Geometry check sheet. Reference: the model listing, model coordinates, mm. A direction names the side the tool comes from. Round coordinates to 2 decimals unless told otherwise and drop trailing zeros. Order: outer loops, then holes, each group sorted by start corner. A loop starts at its lowest first (then second) coordinate and runs counter-clockwise, first axis right, second up. Notation, with made-up numbers: M 20,6 L 74,6 A32 ccw 74,44 Z; hole C 76,67.5 d5. An arc over 180 degrees is marked long. Return JSON: item names as keys, results as strings. Group by question number.
Autodesk Inventor part; units mm, degrees
ref_plane "XZ Plane" through (0, 0, 0) normal (0, 1, 0) x (-1, 0, 0)
ref_plane "XY Plane" through (0, 0, 0) normal (0, 0, 1) x (1, 0, 0)
sketch "Náčrt1" plane through (0, 0, 0) normal (0, 0, 1) x (1, 0, 0)
  line L0 (0, 19.6) -> (0, -19.6)
  line L1 (-19.6, 0) -> (19.6, 0)
  circle A0 centre (0, 0) radius 14
  dimension "d0" = 28
extrude "Vysunutí1" add sketch "Náčrt1" along normal blind 19.2
fillet "Zaoblení1" radius 1 1 edges at (-14, 0, 19.2)
sketch "Náčrt2" plane through (0, 0, 0) normal (0, 0, -1) x (-1, 0, 0)
  line L0 (-7.25, 11) -> (7.25, 11)
  line L1 (7.25, 11) -> (7.25, 17)
  line L2 (7.25, 17) -> (-7.25, 17)
  line L3 (-7.25, 17) -> (-7.25, 11)
  circle A0 centre (0, 0) radius 14
  line L4 (-7.25, 11) -> (7.25, 17) construction
  line L5 (7.25, 11) -> (-7.25, 17) construction
  circle A1 centre (0, 0) radius 15.5
  line L6 (-8.6, 12.8953) -> (-8.6, 11.0472)
  line L7 (8.6, 12.8953) -> (8.6, 11.0472)
  point P0 (0, 14)
  point P1 (0, 14)
  point P2 (7.25, 13.6999)
  point P3 (-7.25, 13.6999)
  dimension "d4" = 14.5
  dimension "d5" = 31
  dimension "d6" = 17.2
  dimension "d7" = 1.35
  dimension "d8" = 1.35
  dimension "d9" = 1.5
extrude "Vysunutí2" add sketch "Náčrt2" against normal blind 16.5 contours A0 L6 A1 L3 | L3 A1 L1 A0 | L1 A1 L7 A0 | L3 L2 L1 A1
sketch "Náčrt3" plane through (0, 0, 0) normal (0, 0, -1) x (-1, 0, 0)
  circle A0 centre (0, -8) radius 4.6
  line L0 (0, -12.6) -> (0, -14) construction
  arc A1 (-8.6, 11.0472) -> (8.6, 11.0472) centre (0, 0) ccw construction
  dimension "d12" = 9.2
  dimension "d14" = 1.4
extrude "Vysunutí3" add sketch "Náčrt3" along normal blind 1.7
sketch "Náčrt4" plane through (0, -8, -1.7) normal (0, 0, -1) x (-1, 0, 0)
  circle A0 centre (0, 0) radius 4.6
  circle A1 centre (0, 0) radius 2.5
  line L0 (-1.475, 2.0185) -> (-1.475, -2.0185)
  line L1 (1.475, 2.0185) -> (1.475, -2.0185)
  point P0 (0, 8)
  dimension "d17" = 5
  dimension "d18" = 2.95
extrude "Vysunutí4" add sketch "Náčrt4" along normal blind 8 contours L1 A1 L0
sketch "Náčrt5" plane through (0, -8, -1.7) normal (0, 0, -1) x (-1, 0, 0)
  arc A0 (1.475, 2.0185) -> (-1.475, 2.0185) centre (0, 0) ccw
  circle A1 centre (0, 0) radius 2.5
  point P0 (0, 8)
  point P1 (-1.475, 2.0185)
  point P2 (1.475, 2.0185)
extrude "Vysunutí5" add sketch "Náčrt5" along normal blind 2
sketch "Sketch6" plane through (0, 0, 0) normal (0, 0, -1) x (-1, 0, 0)
  line L0 (-17.5, 0) -> (17.5, 0) construction
  line L1 (-17.5, -3.5) -> (17.5, -3.5)
  line L2 (17.5, 3.5) -> (-17.5, 3.5)
  arc A0 (-17.5, 3.5) -> (-17.5, -3.5) centre (-17.5, 0) ccw
  arc A1 (17.5, -3.5) -> (17.5, 3.5) centre (17.5, 0) ccw
  circle A2 centre (-17.5, 0) radius 2.1
  circle A3 centre (17.5, 0) radius 2.1
  point P0 (0, 0)
  dimension "d23" = 4.2
  dimension "d24" = 35
  dimension "d25" = 7
extrude "Extrusion6" add sketch "Sketch6" against normal blind 1
equation "\"d7\" = d8"
properties part number "Motor"
Q1. Section check B-B on z = 0.5. Record the cut outline in (x, y), plus the area to 3 significant figures.
Q2. Set-up check for faces 1 (the face through (15.6, -3.5, 0.5)), 2 (the face through (-15.6, 3.5, 0.5)), 3 (the face through (2, -8, -3.7)), 4 (the face through (-1.34, -10.11, -4.76)), 5 (the face through (8.6, 12, 8)): record each of +Z, -Z, +X, -X, +Y, -Y from which the full face is reachable in a straight line by a thin tool's end or side.
Q3. Material ranges on line 1 along Y through (x, z) = (17.5, 0.7); line 2 along X through (y, z) = (-10, -4.5) (3 decimals); line 3 along Z through (x, y) = (2.5, -2), recorded low to high.
Q4. Section check C-C on x = 0. Record the cut outline in (y, z), plus the area to 3 significant figures.
Q5. Section check A-A on y = 0. Record the cut outline in (x, z).
Q6. Section check D-D on z = 17.25. Record the cut outline in (x, y).
Q7. Depth check by flat-ended pin: pin 1 Ø1.2 at (y, z) = (-9, -7) entering from -X (3 decimals); pin 2 Ø12 at (y, z) = (8, 2) entering from +X; pin 3 Ø4.5 at (y, z) = (-8.5, -7) entering from +X (3 decimals); pin 4 Ø1 at (x, z) = (5.5, -1.5) entering from -Y. Enter the tip coordinate at first touch or a pass-through.
Geometry check:
{
 "1": {"outline": "M -17.5,-3.5 L -13.56,-3.5 A14 ccw 13.56,-3.5 L 17.5,-3.5 A3.5 ccw 17.5,3.5 L 13.56,3.5 A14 ccw 8.6,11.05 L 8.6,12.9 A15.5 ccw 7.25,13.7 L 7.25,17 L -7.25,17 L -7.25,13.7 A15.5 ccw -8.6,12.9 L -8.6,11.05 A14 ccw -13.56,3.5 L -17.5,3.5 A3.5 ccw Z; hole C -17.5,0 d4.2; hole C 17.5,0 d4.2", "area": "735 mm^2"},
 "2": {"face 1": "+Z, -Z, +X, -Y", "face 2": "+Z, -Z, -X, +Y", "face 3": "-Z, +X, +Y, -Y", "face 4": "-Z", "face 5": "+Z, -Z, +X, +Y"},
 "3": {"line 1": "y = -3.5 to -2.1, 2.1 to 3.5", "line 2": "x = -1.475 to 1.475", "line 3": "z = 0 to 19.2"},
 "4": {"outline": "M -14,0 L -12.6,0 L -12.6,-1.7 L -10.5,-1.7 L -10.5,-9.7 L -5.5,-9.7 L -5.5,-1.7 L -3.4,-1.7 L -3.4,0 L 17,0 L 17,16.5 L 14,16.5 L 14,18.2 A1 ccw 13,19.2 L -13,19.2 A1 ccw -14,18.2 Z", "area": "642 mm^2"},
 "5": {"outline": "M -21,0 L -19.6,0 L -19.6,1 L -21,1 Z; M -15.4,0 L 15.4,0 L 15.4,1 L 14,1 L 14,18.2 A1 ccw 13,19.2 L -13,19.2 A1 ccw -14,18.2 L -14,1 L -15.4,1 Z; M 19.6,0 L 21,0 L 21,1 L 19.6,1 Z"},
 "6": {"outline": "C 0,0 d28"},
 "7": {"pin 1": "stops at x = -1.475", "pin 2": "stops at x = 20.31", "pin 3": "stops at x = 1.475", "pin 4": "passes through"}
}
